Read the model definition and answer for the solid it produces. Units are mm, in the model's axes. A direction names the side the tool comes from. Round coordinates to 2 decimals unless told otherwise and drop trailing zeros. Write each loop counter-clockwise with the first axis right and the second up, starting at its lowest first coordinate (ties: lowest second). Pieces come first, ordered by that corner, then holes. Notation, with made-up numbers: (84.25, 37.5) -> (128.25, 37.5) arc R29 cw to (128.25, 65.5) -> close; hole circle Ø5 at (24, 37). An arc over 180 degrees is marked (long way). Return JSON: item names as keys, results as strings.
from build123d import *

# Parameters (mm, degrees)
SKETCH1_W                    = 103
SKETCH1_H                    = 68
BOSS_EXTRUDE1_DEPTH          = 30
SKETCH2_W                    = 92.99558251
SKETCH2_H                    = 57.998770124
CUT_EXTRUDE1_DEPTH           = 28
SKETCH3_W                    = 7.71242133
SKETCH3_H                    = 22.765769716
CUT_EXTRUDE2_DEPTH           = 28
F_97_0_0059_DIAMETER_HOLE1_D = 0.14986


with BuildPart() as part:
    # Sketch1 → Boss-Extrude1 (new body)
    with BuildSketch(Plane(origin=(0, 0, 0), x_dir=(1, 0, 0), z_dir=(0, 1, 0))):
        with Locations((-0.5, 0.75)):
            Rectangle(SKETCH1_W, SKETCH1_H)
    extrude(amount=BOSS_EXTRUDE1_DEPTH)

    # Sketch2 → Cut-Extrude1 (cut)
    with BuildSketch(Plane(origin=(51, 30, -34.75), x_dir=(1, 0, 0), z_dir=(0, -1, 0))):
        with Locations((-51.502635722, 33.995679306)):
            Rectangle(SKETCH2_W, SKETCH2_H)
    extrude(amount=CUT_EXTRUDE1_DEPTH, mode=Mode.SUBTRACT)

    # Sketch3 → Cut-Extrude2 (cut)
    with BuildSketch(Plane(origin=(51, 0, 0), x_dir=(0, 0, -1), z_dir=(1, 0, 0))):
        with Locations((-24.383198114, 18.617115142)):
            Rectangle(SKETCH3_W, SKETCH3_H)
    extrude(amount=-CUT_EXTRUDE2_DEPTH, mode=Mode.SUBTRACT)

    # #97 (0.0059) Diameter Hole1 (through all)
    with Locations(Plane(origin=(0, 30, 0), x_dir=(1, 0, 0), z_dir=(0, 1, 0))):
        with Locations((49.13026129, -30.550335592), (49.13026129, 32.624025804), (-49.65125644, 32.624025804), (-49.65125644, -30.550335592)):
            Hole(F_97_0_0059_DIAMETER_HOLE1_D / 2)


solid = part.part
Item 1: Flat-ended cylindrical pins translate along their axes: pin 1 (1.5 mm diameter, centred on x = 48.5, z = 25, fed in from +Y); pin 2 (8 mm diameter, centred on x = 18, z = -13, fed in from +Y); pin 3 (10 mm diameter, centred on x = 23.5, z = -18.5, fed in from -Y). Find the tip coordinate at first contact, or state that the pin passes through.
Worked answers:
{"pin 1": "stops at y = 7.23", "pin 2": "stops at y = 2", "pin 3": "stops at y = 0"}
Item 2: For a pull along X with two mould halves and no side action, classify faces 1 (the flat face through (51, 15, 0)), 2 (the flat face through (49, 18, 20.527)), 3 (the flat face through (-1, 16, 28.245)) as released by +X, released by -X, zero draft, split by the parting line, or undercut.
Worked answers:
{"face 1": "released by +X", "face 2": "zero draft", "face 3": "undercut"}
Item 3: Section D-D (y = 15.25) is taken. State how many separate pieces and enclosed holes the cut face has, then the cut area to 3 significant figures.
Worked answers:
{"separate pieces": "1", "enclosed holes": "4", "area": "1,570 mm2"}
Item 4: A tool of negligible diameter and unlimited length cuts with its end or side. For faces 4 (the flat face through (-52, 15, 0)), 5 (the flat face through (-47, 16, -1)), 6 (the flat face through (49, 7.234, 24)), from which of +Z, -Z, +X, -X, +Y, -Y can it reach the whole face along a straight path? Write none if from no direction.
Worked answers:
{"face 4": "+Z, -Z, -X, +Y, -Y", "face 5": "+Y", "face 6": "+X, +Y"}
Item 5: Section C-C (x = -31) is taken. Give the vertices of the cut face in (y, z).
Worked answers:
{"outline": "(0, -34.75) -> (30, -34.75) -> (30, -29.75) -> (2, -29.75) -> (2, 28.25) -> (30, 28.25) -> (30, 33.25) -> (0, 33.25) -> close"}
Item 6: Straight lines are drawn through the part: L1, parallel to Z at x = -25.5, y = 5.75; L2, parallel to X at y = 3.5, z = 8.5; L3, parallel to Y at x = -23, z = 17.5. For each, find the intervals that lie inside material, in ascending order. Write a range as [from, to].
Worked answers:
{"L1": "z = [-34.75, -29.75], [28.25, 33.25]", "L2": "x = [-52, -47], [46, 51]", "L3": "y = [0, 2]"}
Item 7: Section B-B (y = 3.75) is taken. Give the vertices of the cut face in (x, z), then the cut area to 3 significant figures.
Worked answers:
{"outline": "(-52, -34.75) -> (51, -34.75) -> (51, 33.25) -> (-52, 33.25) -> close; hole circle Ø0.15 at (-49.65, -32.62); hole circle Ø0.15 at (-49.65, 30.55); hole (-47, -29.75) -> (46, -29.75) -> (46, 28.25) -> (-47, 28.25) -> close; hole circle Ø0.15 at (49.13, -32.62); hole circle Ø0.15 at (49.13, 30.55)", "area": "1,610 mm2"}
Item 8: Section A-A (z = -20) is taken. Give the vertices of the cut face in (x, y).
Worked answers:
{"outline": "(-52, 0) -> (51, 0) -> (51, 30) -> (46, 30) -> (46, 2) -> (-47, 2) -> (-47, 30) -> (-52, 30) -> close"}
